The figure shows three views and two pictorial views of one solid part (mm, origin at its lowest corner). Answer the questions. Coordinates: 2 decimals unless noted, no trailing zeros. Order: outer loops, then holes, each group sorted by start corner. A loop starts at its lowest first (then second) coordinate and runs counter-clockwise, first axis right, second up. Notation, with made-up numbers: (33, 51.25) -> (47, 51.25) arc R30 ccw to (47, 78.25) -> close; hole circle Ø6 at (25.25, 79.25). An arc over 180 degrees is marked (long way). Use one line per item in the form item = value.
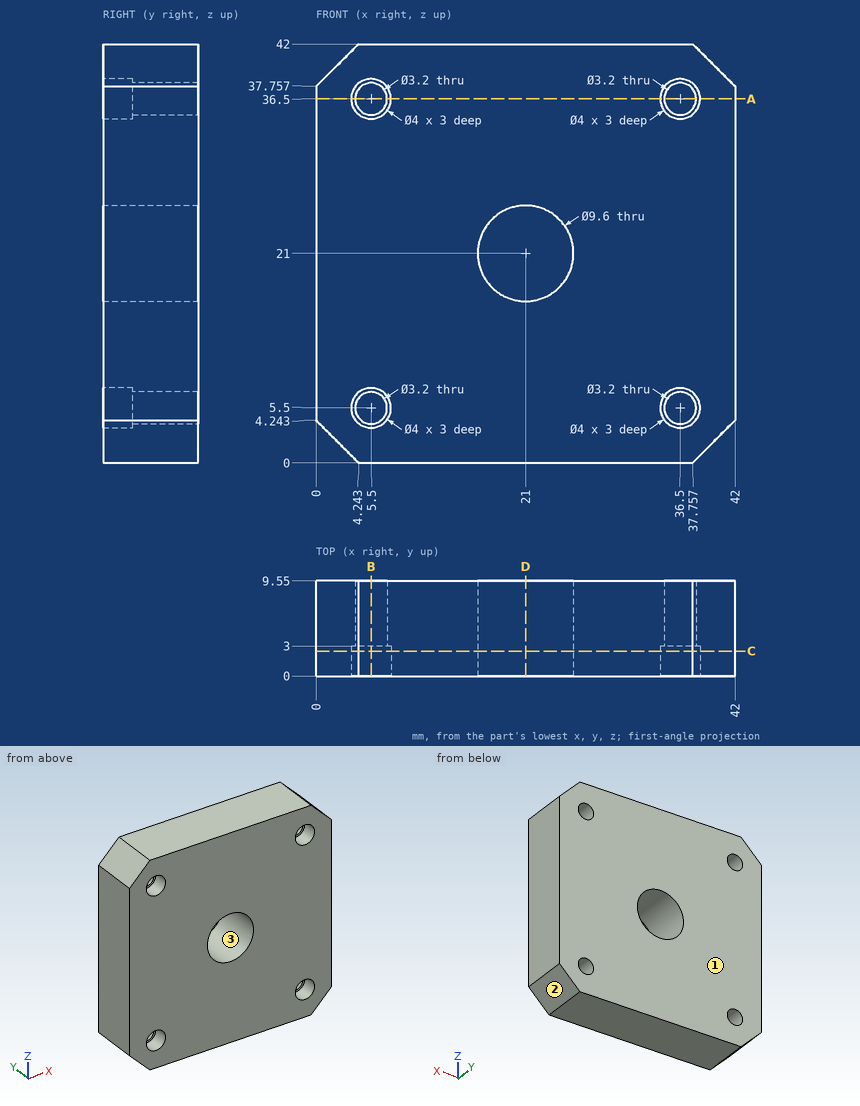
(1) Straight lines are drawn through the part: line 1 along X through (y, z) = (5, 36.5); line 2 along X through (y, z) = (6.25, 21); line 3 along X through (y, z) = (8.25, 17.5) (1 decimal). For each, find the intervals that lie inside material, in ascending order.
Data:
line_1 = 0 to 3.9, 7.1 to 34.9, 38.1 to 42
line_2 = 0 to 16.2, 25.8 to 42
line_3 = 0 to 17.7, 24.3 to 42
(2) The mould has two halves that part along X. Classify the marked faces 1, 2 and 3: released by +X, released by -X, zero draft, split by the parting line, or undercut.
Data:
face_1 = zero draft
face_2 = released by +X
face_3 = undercut
(3) Section D-D on x = 21 is taken. Write down the section's boundary in (y, z).
Data:
outline = (0, 0) -> (9.55, 0) -> (9.55, 16.2) -> (0, 16.2) -> close; (0, 25.8) -> (9.55, 25.8) -> (9.55, 42) -> (0, 42) -> close
(4) Section C-C on y = 2.5 is taken. Write down the section's boundary in (x, z).
Data:
outline = (0, 4.24) -> (4.24, 0) -> (37.76, 0) -> (42, 4.24) -> (42, 37.76) -> (37.76, 42) -> (4.24, 42) -> (0, 37.76) -> close; hole circle Ø4 at (5.5, 5.5); hole circle Ø4 at (5.5, 36.5); hole circle Ø9.6 at (21, 21); hole circle Ø4 at (36.5, 5.5); hole circle Ø4 at (36.5, 36.5)
(5) Each of these flat-tipped pins is pushed along its axis until it touches: P1, Ø1.2, axis at x = 5, z = 6.5, coming from the -Y side; P2, Ø3, axis at x = 5.5, z = 36.5, coming from the +Y side. Where does it stop, or does it pass through?
Data:
P1 = 3
P2 = through
(6) Section B-B on x = 5.5 is taken. Write down the section's boundary in (y, z), plus the area to 3 significant figures.
Data:
outline = (0, 0) -> (9.55, 0) -> (9.55, 3.9) -> (3, 3.9) -> (3, 3.5) -> (0, 3.5) -> close; (0, 7.5) -> (3, 7.5) -> (3, 7.1) -> (9.55, 7.1) -> (9.55, 34.9) -> (3, 34.9) -> (3, 34.5) -> (0, 34.5) -> close; (0, 38.5) -> (3, 38.5) -> (3, 38.1) -> (9.55, 38.1) -> (9.55, 42) -> (0, 42) -> close
area = 335 mm²
(7) Section A-A on z = 36.5 is taken. Write down the section's boundary in (x, y), plus the area to 3 significant figures.
Data:
outline = (0, 0) -> (3.5, 0) -> (3.5, 3) -> (3.9, 3) -> (3.9, 9.55) -> (0, 9.55) -> close; (7.1, 3) -> (7.5, 3) -> (7.5, 0) -> (34.5, 0) -> (34.5, 3) -> (34.9, 3) -> (34.9, 9.55) -> (7.1, 9.55) -> close; (38.1, 3) -> (38.5, 3) -> (38.5, 0) -> (42, 0) -> (42, 9.55) -> (38.1, 9.55) -> close
area = 335 mm²
